from build123d import *

# Parameters (mm, degrees)
F0_W   = 41.94641
F0_H   = 26.064575
F0_W_2 = 42.390289
F0_H_2 = 29.70939


with BuildPart() as f1:
    # F0 (on Front) → F1 (revolve)
    with BuildSketch(Plane.XZ):
        with Locations((-37.19489, -6.956225)):
            Rectangle(F0_W, F0_H)
    revolve(axis=Axis((67.449205, 0, -2.508159), (0, 0, -1)))


with BuildPart() as f2:
    # F0 (on Front) → F2 (revolve)
    with BuildSketch(Plane.XZ):
        with Locations((46.25406, -2.508159)):
            Rectangle(F0_W_2, F0_H_2)
    revolve(axis=Axis((-58.168095, 0, -6.956225), (0, 0, -1)))


with BuildPart() as f1_1:
    add(f1.part)

    # F3: cut F2
    add(f2.part, mode=Mode.SUBTRACT)


solid = f1_1.part
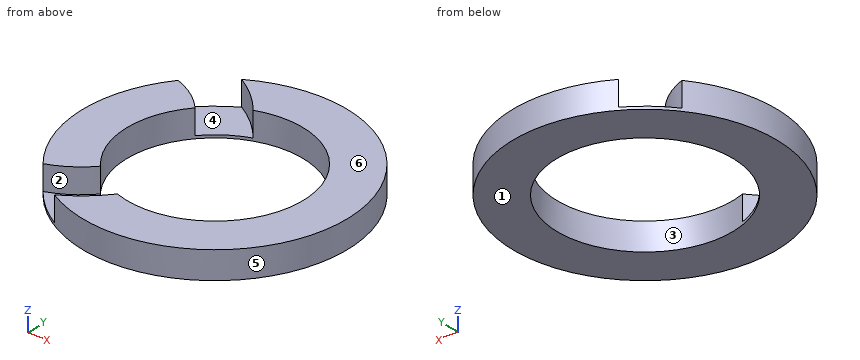
Source: CAD feature listing. Evaluate the final solid. Frame: model axes, mm. Face numbers are marked on the shaded views. A direction names the side the tool comes from. Round coordinates to 2 decimals unless told otherwise and drop trailing zeros. Loops run counter-clockwise (first coordinate to the right, second up) from the corner with the lowest first, then second, coordinate; pieces in that order, holes last. Notation, with made-up numbers: (78.5, 36) -> (94.5, 36) arc R24 cw to (94.5, 62) -> close; hole circle Ø6 at (59.5, 60.25). An arc over 180 degrees is marked (long way). Answer as a JSON object with one key per item and string values. Group by question number.
Q1. Section query C-C (y = -90.5). Output: boundary loops of the cut face in (x, z), plus the area to 3 significant figures.
Q2. Section query D-D (y = 74.5). Output: boundary loops of the cut face in (x, z).
Q3. Section query A-A (y = 0). Output: boundary loops of the cut face in (x, z), plus the area to 3 significant figures.
Q4. Mould query, pull axis Y, two halves, no side actions, for the marked faces 3, 4, 5 and 6. Classes: pulls with the +Y half, pulls with the -Y half, needs draft (parallel to the pull), parting line crosses it, or undercut.
Q5. Contact query for flat-ended pins moving along their axis: P1, Ø6, axis at y = 30.5, z = -17.5, coming from the +X side; P2, Ø12, axis at y = -24.5, z = -3.5, coming from the -X side; P3, Ø12, axis at y = -41.5, z = -2.5, coming from the +X side. Output: stop coordinate, or through.
Q6. Access query for the marked faces 1 and 2. Directions: +Z, -Z, +X, -X, +Y, -Y. A direction counts if a zero-diameter tool reaches every point of the face in a straight line with its end or side. Return the directions, or none.
Q7. Section query B-B (z = 0). Output: boundary loops of the cut face in (x, y), plus the area to 3 significant figures.
Q8. Ray query, line 1 (Y direction, x = 132, z = -12.5); line 2 (X direction, y = -67.5, z = -7.5); line 3 (X direction, y = -56, z = -13). Return the intervals inside material, ascending. Write a range as from..to.
Completed:
{
 "1": {"outline": "(-19.67, -19.99) -> (154.57, -19.99) -> (154.57, 6.08) -> (28.95, 6.08) -> (28.95, -17.36) -> (-19.67, -17.36) -> close", "area": "3,400 mm²"},
 "2": {"outline": "(-33.69, -19.99) -> (29.36, -19.99) -> (29.36, -17.36) -> (-21.07, -17.36) -> (-21.07, 6.08) -> (-33.69, 6.08) -> close; (105.54, -19.99) -> (168.59, -19.99) -> (168.59, 6.08) -> (105.54, 6.08) -> close"},
 "3": {"outline": "(-58.17, -19.99) -> (-16.22, -19.99) -> (-16.22, 6.08) -> (-58.17, 6.08) -> close; (151.12, -19.99) -> (193.07, -19.99) -> (193.07, 6.08) -> (151.12, 6.08) -> close", "area": "2,190 mm²"},
 "4": {"face 3": "undercut", "face 4": "undercut", "face 5": "parting line crosses it", "face 6": "needs draft"},
 "5": {"P1": "x = 190.02", "P2": "x = -56.8", "P3": "x = 187.95"},
 "6": {"face 1": "-Z, +X, -X, +Y, -Y", "face 2": "+Z, -Y"},
 "7": {"outline": "(-30.6, -78.53) arc R83.23 ccw to (4.35, -54.94) arc R83.67 cw to (4.35, 54.94) arc R83.23 ccw to (-30.6, 78.53) arc R125.62 ccw to start; (4.64, -108.79) arc R125.62 ccw (long way) to (4.64, 108.79) arc R125.62 cw to (39.58, 78.89) arc R83.67 cw (long way) to (39.58, -78.89) arc R125.62 cw to start", "area": "23,800 mm²"},
 "8": {"line 1": "-107.76..-53.24, 53.24..107.76", "line 2": "-38.49..-9.48, 116.89..173.39", "line 3": "-45..3.4, 129.62..179.89"}
}
